from build123d import *

# Parameters (mm, degrees)
SKETCH1_W           = 40
SKETCH1_H           = 25
BOSS_EXTRUDE1_DEPTH = 5
SKETCH6_R           = 18
SKETCH6_R_2         = 3
BOSS_EXTRUDE4_DEPTH = 5
SKETCH7_W           = 25
SKETCH7_H           = 25
BOSS_EXTRUDE5_DEPTH = 5


with BuildPart() as part:
    # Sketch1 → Boss-Extrude1 (new body)
    with BuildSketch(Plane(origin=(0, 0, 0), x_dir=(1, 0, 0), z_dir=(0, 1, 0))):
        with Locations((20, 0)):
            Rectangle(SKETCH1_W, SKETCH1_H)
    boss_extrude1 = extrude(amount=BOSS_EXTRUDE1_DEPTH)

    # Sketch6 → Boss-Extrude4 (add)
    # profile 1 of 2: a face of its own
    with BuildSketch(Plane(origin=(40, 0, 0), x_dir=(0, 0, -1), z_dir=(1, 0, 0))):
        with Locations((0, 30)):
            Circle(SKETCH6_R)
        with Locations((0, 30)):
            Circle(SKETCH6_R_2, mode=Mode.SUBTRACT)
    # profile 2 of 2: a face of its own
    with BuildSketch(Plane(origin=(40, 0, 0), x_dir=(0, 0, -1), z_dir=(1, 0, 0))):
        with BuildLine():
            ThreePointArc((12.5, 17.048166153), (0, 12), (-12.5, 17.048166153))
            Line((-12.5, 17.048166153), (-12.5, 5))
            Line((-12.5, 5), (12.5, 5))
            Line((12.5, 5), (12.5, 17.048166153))
        make_face()
    boss_extrude4 = extrude(amount=-BOSS_EXTRUDE4_DEPTH)

    # Mirror2: Boss-Extrude1, Boss-Extrude4 across plane
    add(boss_extrude1.mirror(Plane(origin=(0, 5, -12.5), x_dir=(0, 0, 1), z_dir=(1, 0, 0))))
    add(boss_extrude4.mirror(Plane(origin=(0, 5, -12.5), x_dir=(0, 0, 1), z_dir=(1, 0, 0))))

    # Sketch7 → Boss-Extrude5 (add)
    with BuildSketch(Plane.XZ):
        Rectangle(SKETCH7_W, SKETCH7_H)
    extrude(amount=BOSS_EXTRUDE5_DEPTH)


solid = part.part
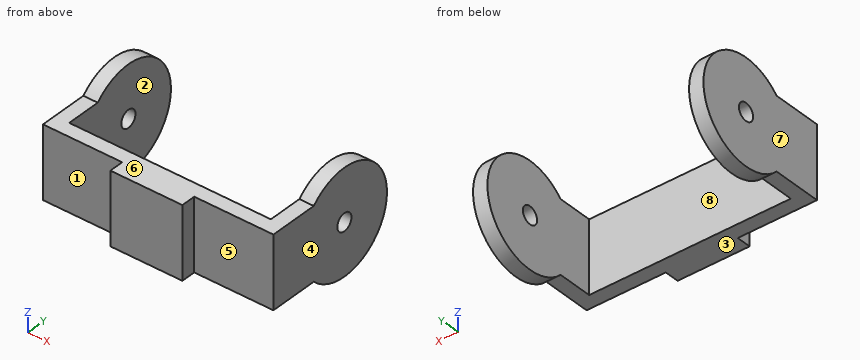
Design review of the part built by this model. Coordinates are the model's own, in mm. Face numbers are marked on the shaded views. A direction names the side the tool comes from. Coordinates: 2 decimals unless noted, no trailing zeros. Write each loop counter-clockwise with the first axis right and the second up, starting at its lowest first coordinate (ties: lowest second). Pieces come first, ordered by that corner, then holes. Notation, with made-up numbers: (-29.75, 25.5) - (6.25, 25.5) arc R24 ccw to (6.25, 37.5) - close; hole circle Ø3 at (86, 48.5). An arc over 180 degrees is marked (long way). One line per item, written item: value.
1) Insertion check: pin 1 (3 mm diameter, centred on x = 15.5, z = 9, fed in from -Y); pin 2 (7 mm diameter, centred on y = 30, z = 0, fed in from -X); pin 3 (17.5 mm diameter, centred on x = -18.5, y = 7, fed in from +Z); pin 4 (7.5 mm diameter, centred on x = -4.5, z = -1.5, fed in from +Y). Each pin has a flat end and moves straight along its axis. Give the tip position at first contact, or say it passes through.
Answer sheet:
pin 1: stops at y = 0
pin 2: stops at x = -40
pin 3: stops at z = 12.5
pin 4: stops at y = 5
2) Add section A-A (y = 6). State the section outline as (x, z) points, plus the area to 3 significant figures.
Answer sheet:
outline: (-40, -12.5) - (-35, -12.5) - (-35, 12.5) - (-40, 12.5) - close; (35, -12.5) - (40, -12.5) - (40, 12.5) - (35, 12.5) - close
area: 250 mm2
3) Add section C-C (y = 30). State the section outline as (x, z) points, plus the area to 3 significant figures.
Answer sheet:
outline: (-40, -18) - (-35, -18) - (-35, -3) - (-40, -3) - close; (-40, 3) - (-35, 3) - (-35, 18) - (-40, 18) - close; (35, -18) - (40, -18) - (40, -3) - (35, -3) - close; (35, 3) - (40, 3) - (40, 18) - (35, 18) - close
area: 300 mm2
4) To check wall thickness, follow probe 1 along X at (y, z) = (31.5, 10); probe 2 along Y at (x, z) = (-38.85, 0); probe 3 along Z at (x, y) = (28, 4.5). State the ranges of each line that lie inside material, in increasing order.
Answer sheet:
probe 1: x = -40 to -35, 35 to 40
probe 2: y = 0 to 27, 33 to 48
probe 3: z = -12.5 to 12.5
5) Add section B-B (z = 0). State the section outline as (x, y) points, plus the area to 3 significant figures.
Answer sheet:
outline: (-40, 0) - (-12.5, 0) - (-12.5, -5) - (12.5, -5) - (12.5, 0) - (40, 0) - (40, 27) - (35, 27) - (35, 5) - (-35, 5) - (-35, 27) - (-40, 27) - close; (-40, 33) - (-35, 33) - (-35, 48) - (-40, 48) - close; (35, 33) - (40, 33) - (40, 48) - (35, 48) - close
area: 895 mm2
6) For the marked faces 1, 2, 3, 4 and 5, list the 3-axis set-ups (+Z, -Z, +X, -X, +Y, -Y) from which the entire face can be reached by the end or side of a thin tool; tool diameter is ignored.
Answer sheet:
face 1: +Z, -Z, -X, -Y
face 2: +Z, -Z, +Y
face 3: -Z, +X, -X, -Y
face 4: +Z, -Z, +X, +Y, -Y
face 5: +Z, -Z, +X, -Y
7) Add section D-D (z = -15.5). State the section outline as (x, y) points, plus the area to 3 significant figures.
Answer sheet:
outline: (-40, 20.85) - (-35, 20.85) - (-35, 39.15) - (-40, 39.15) - close; (35, 20.85) - (40, 20.85) - (40, 39.15) - (35, 39.15) - close
area: 183 mm2
8) Mouldability with a two-part tool opening along X and no side actions: class the marked faces 6, 7 and 8 as +X half, -X half, draft (parallel to the pull), parting line (faces both ways), or undercut.
Answer sheet:
face 6: draft
face 7: -X half
face 8: undercut
